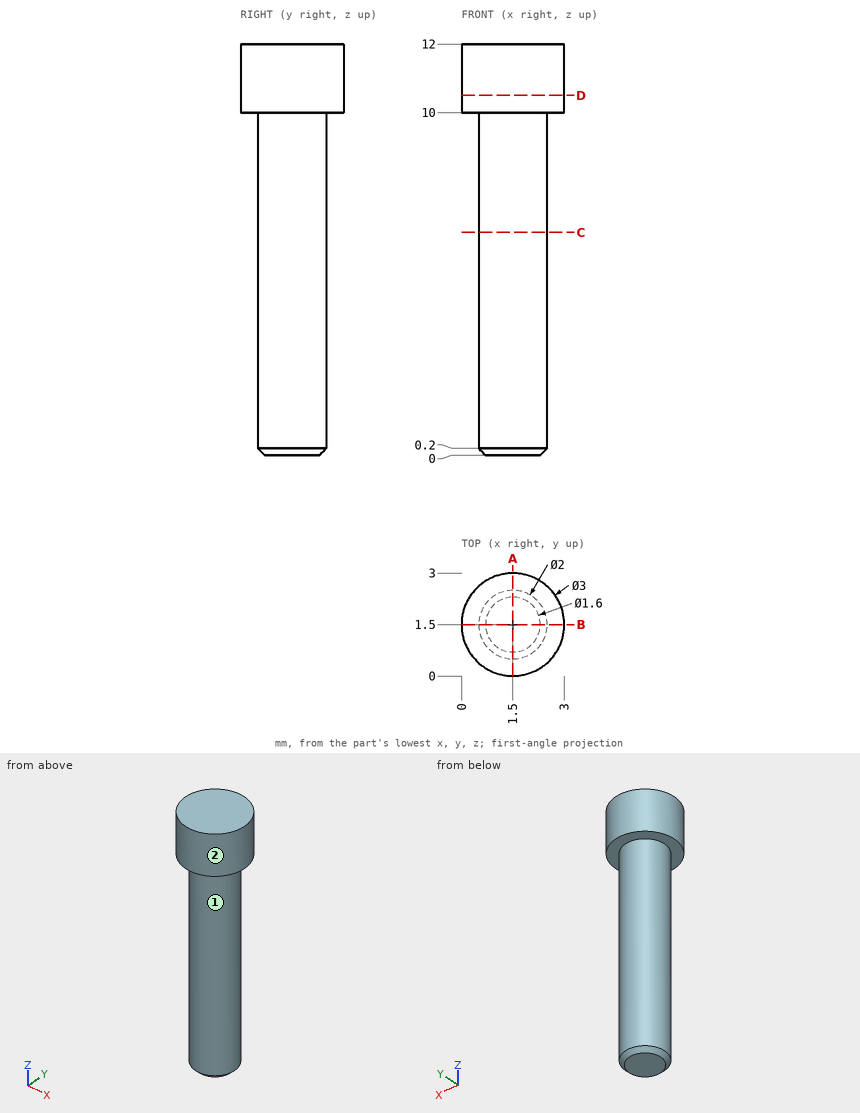
Design review of the part shown in the three views and the two pictorial views. Dimensions are in mm from the part's minimum x, y and z. A direction names the side the tool comes from. Coordinates: 2 decimals unless noted, no trailing zeros. Write each loop counter-clockwise with the first axis right and the second up, starting at its lowest first coordinate (ties: lowest second). Pieces come first, ordered by that corner, then holes.
(1) Tool access review of the marked faces 1 and 2: name each direction out of +Z, -Z, +X, -X, +Y, -Y from which nothing blocks a thin tool from reaching the whole face with its end or side.
(2) Add section D-D on z = 10.5. Give the boundary of the cut face in (x, y).
(3) Add section A-A on x = 1.5. Give the boundary of the cut face in (y, z), then the cut area to 3 significant figures.
(4) Wall thickness on probe 1 along Z at (x, y) = (2.05, 2.6); probe 2 along X at (y, z) = (1.55, 4.75); probe 3 along X at (y, z) = (2.25, 3.5): over which ranges is each line inside the solid? List them lowest first.
(5) For pin 1 Ø1.5 at (x, y) = (2, 1.5) entering from -Z, flat-tipped, find the tip position at first contact; note if it passes through.
(6) Add section C-C on z = 6.5. Give the boundary of the cut face in (x, y), then the cut area to 3 significant figures.
Answer sheet:
1. face 1: -Z
1. face 2: +Z, -Z
2. outline: circle Ø3 at (1.5, 1.5)
3. outline: (0, 10) - (0.5, 10) - (0.5, 0.2) - (0.7, 0) - (2.3, 0) - (2.5, 0.2) - (2.5, 10) - (3, 10) - (3, 12) - (0, 12) - close
3. area: 26.0 mm2
4. probe 1: z = 10 to 12
4. probe 2: x = 0.5 to 2.5
4. probe 3: x = 0.84 to 2.16
5. pin 1: stops at z = 0
6. outline: circle Ø2 at (1.5, 1.5)
6. area: 3.14 mm2
